Here's the drawing with two shaded views (mm, measured from the low corner). I have some questions. A direction names the side the tool comes from. Give positions to 0.01 mm unless a question says otherwise; leave off trailing zeros. Loops run counter-clockwise (first coordinate to the right, second up) from the corner with the lowest first, then second, coordinate; pieces in that order, holes last. Notation, with made-up numbers: M 39,3.5 L 44,3.5 A12 cw 44,8.5 Z; hole C -11,32 d1. An arc over 180 degrees is marked long. Use a Markdown table: item, result. Add a question column.
1) Suppose I cut it at A-A on x = 14.5. List the corners of the cut face in (y, z) for me (1 decimal), and give its area (3 significant figures).
2) Suppose I cut it at C-C on y = 3.2. List the corners of the cut face in (x, z) for me (1 decimal), and give its area (3 significant figures).
3) Will these pins go through, and if not, where does the flat tip stop? pin 1 Ø1.3 at (x, y) = (4.5, 2) entering from -Z; pin 2 Ø3 at (y, z) = (3.5, 53.5) entering from -X; pin 3 Ø3 at (x, y) = (5, 2) entering from +Z; pin 4 Ø18 at (x, z) = (18.92, 27.81) entering from -Y.
4) Suppose I cut it at D-D on z = 12. List the corners of the cut face in (x, y) for me.
5) If I drill on line 1 along Z through (x, y) = (19, 3.9) (1 decimal); line 2 along X through (y, z) = (3.35, 24) (1 decimal); line 3 along X through (y, z) = (0.3, 37.5) (1 decimal), over which ranges is the centre line in solid material (lowest first)? Write a range as [from, to].
6) Which directions (+Z, -Z, +X, -X, +Y, -Y) give clear straight access to the entire face, cutting with the end or side of a thin tool? Please do the marked faces 1, 2 and 3.
7) Suppose I cut it at B-B on z = 23. List the corners of the cut face in (x, y) for me (1 decimal).
8) We'd pull the mould along Z, two halves only. Please class the marked faces 4, 5, 6 and 7: +Z half, -Z half, draft (parallel to the pull), parting line (faces both ways), or undercut.
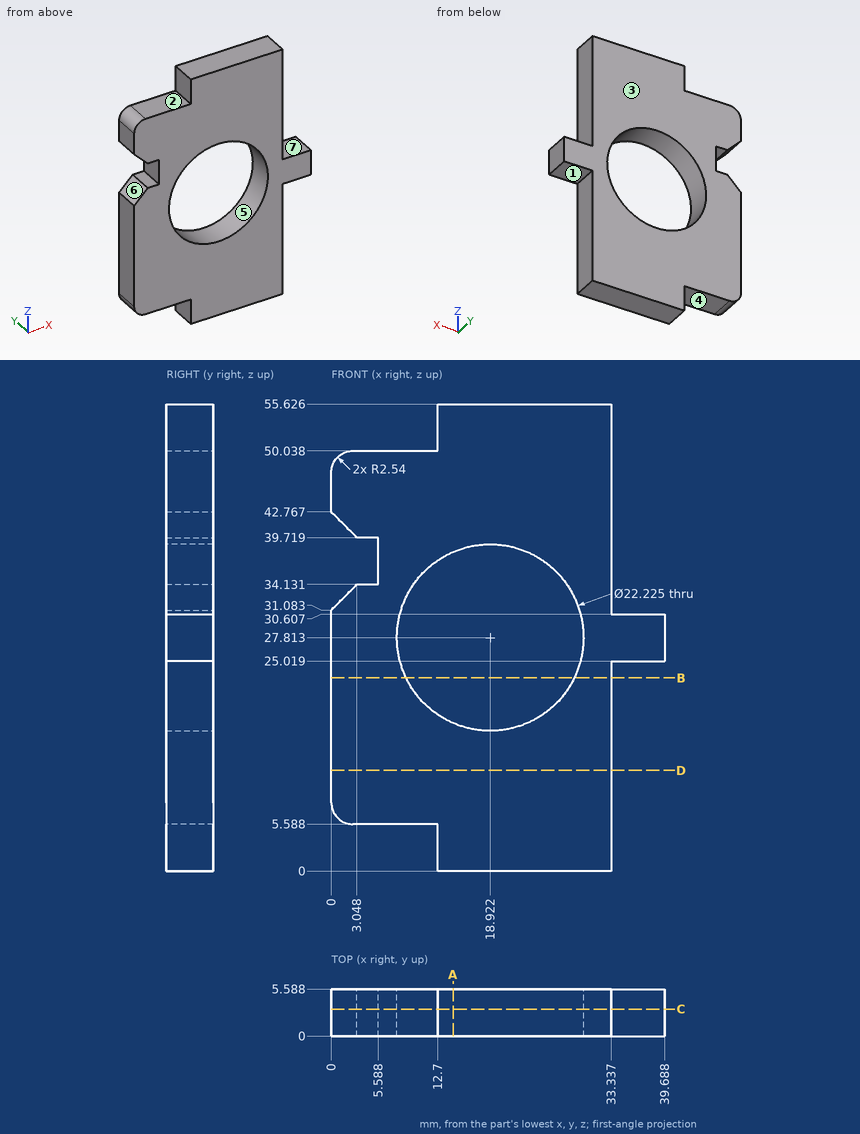
Answer block:
| question | item | result |
|---|---|---|
| 1 | outline | M 0,0 L 5.6,0 L 5.6,17.6 L 0,17.6 Z; M 0,38 L 5.6,38 L 5.6,55.6 L 0,55.6 Z |
| 1 | area | 197 mm^2 |
| 2 | outline | M 0,8.1 A2.5 ccw 2.5,5.6 L 12.7,5.6 L 12.7,0 L 33.3,0 L 33.3,25 L 39.7,25 L 39.7,30.6 L 33.3,30.6 L 33.3,55.6 L 12.7,55.6 L 12.7,50 L 2.5,50 A2.5 ccw 0,47.5 L 0,42.8 L 3,39.7 L 5.6,39.7 L 5.6,34.1 L 3,34.1 L 0,31.1 Z; hole C 18.9,27.8 d22.2 |
| 2 | area | 1,320 mm^2 |
| 3 | pin 1 | stops at z = 5.59 |
| 3 | pin 2 | stops at x = 12.7 |
| 3 | pin 3 | stops at z = 50.04 |
| 3 | pin 4 | passes through |
| 4 | outline | M 0,0 L 33.34,0 L 33.34,5.59 L 0,5.59 Z |
| 5 | line 1 | z = [0, 16.7], [38.9, 55.6] |
| 5 | line 2 | x = [0, 8.5], [29.4, 33.3] |
| 5 | line 3 | x = [5.6, 13.5], [24.4, 33.3] |
| 6 | face 1 | -Z, +X, +Y, -Y |
| 6 | face 2 | +Z, -X, +Y, -Y |
| 6 | face 3 | +Z, -Z, +X, -X, +Y |
| 7 | outline | M 0,0 L 8.9,0 L 8.9,5.6 L 0,5.6 Z; M 28.9,0 L 33.3,0 L 33.3,5.6 L 28.9,5.6 Z |
| 8 | face 4 | -Z half |
| 8 | face 5 | undercut |
| 8 | face 6 | undercut |
| 8 | face 7 | +Z half |
